CAD build for the part. Positions are in the model's coordinates, mm. Give positions to 0.01 mm unless a question says otherwise; leave off trailing zeros. Write each loop counter-clockwise with the first axis right and the second up, starting at its lowest first coordinate (ties: lowest second). Pieces come first, ordered by that corner, then holes. Notation, with made-up numbers: (44, -35) - (85, -35) arc R21 cw to (85, -14) - close; hole circle Ø10 at (87.25, 88). An arc over 180 degrees is marked (long way). Answer as a JSON object with one key per item and string values.
Autodesk Inventor part; units mm, degrees
ref_plane "XZ Plane" through (0, 0, 0) normal (0, 1, 0) x (-1, 0, 0)
ref_plane "XY Plane" through (0, 0, 0) normal (0, 0, 1) x (1, 0, 0)
sketch "Sketch1" plane through (0, 0, 0) normal (0, 1, 0) x (-1, 0, 0)
  line L0 (0, 0) -> (0, -399.562) construction
  line L1 (5, 0) -> (5, -399.562)
  line L2 (-5, -399.562) -> (-5, 0)
  arc A0 (5, 0) -> (-5, 0) centre (0, 0) ccw
  arc A1 (-5, -399.562) -> (5, -399.562) centre (0, -399.562) ccw
  circle A2 centre (0, -399.562) radius 1.65
  line L3 (0, -10) -> (0, -379.562) construction
  line L4 (-1.65, -10) -> (-1.65, -379.562)
  line L5 (1.65, -379.562) -> (1.65, -10)
  arc A3 (1.65, -10) -> (-1.65, -10) centre (0, -10) ccw
  arc A4 (-1.65, -379.562) -> (1.65, -379.562) centre (0, -379.562) ccw
  point P0 (0, -199.781)
  point P1 (0, -194.781)
  dimension "d1" = 3.3
  dimension "d2" = 10
  dimension "d3" = 399.562
  dimension "d16" = 3.3
  dimension "d17" = 20
  dimension "d18" = 10
extrude "Extrusion1" add sketch "Sketch1" along normal blind 6
sketch "Sketch2" plane through (0, 6, 0) normal (0, 1, 0) x (1, 0, 0)
  line L0 (-5, 399.562) -> (-5, 0)
  arc A0 (-5, 0) -> (5, 0) centre (0, 0) ccw
  line L1 (5, 0) -> (5, 399.562)
  arc A1 (5, 399.562) -> (-5, 399.562) centre (0, 399.562) ccw
  arc A2 (-1.65, 10) -> (1.65, 10) centre (0, 10) ccw
  line L2 (-1.65, 10) -> (-1.65, 379.562)
  arc A3 (1.65, 379.562) -> (-1.65, 379.562) centre (0, 379.562) ccw
  line L3 (1.65, 379.562) -> (1.65, 10)
  circle A4 centre (0, 399.562) radius 1.65
  line L4 (-5, 399.562) -> (-5, 0)
  line L5 (5, 0) -> (5, 399.562)
  circle A5 centre (0, 384.562) radius 5
  point P0 (-5, 384.562)
  point P1 (5, 384.562)
  dimension "d20" = 15
  dimension "d21" = 10
extrude "Extrusion2" add sketch "Sketch2" along normal blind 4 contours A1 L1 A5 L0 | A5 A3 | A3 A5
sketch "Sketch3" plane through (0, 0, 0) normal (0, -1, 0) x (1, 0, 0)
  line L0 (-5, -399.562) -> (-5, 0)
  arc A0 (-5, -399.562) -> (5, -399.562) centre (0, -399.562) ccw
  line L1 (5, 0) -> (5, -399.562)
  arc A1 (5, 0) -> (-5, 0) centre (0, 0) ccw
  arc A2 (1.65, -10) -> (-1.65, -10) centre (0, -10) ccw
  line L2 (1.65, -379.562) -> (1.65, -10)
  arc A3 (-1.65, -379.562) -> (1.65, -379.562) centre (0, -379.562) ccw
  line L3 (-1.65, -10) -> (-1.65, -379.562)
  circle A4 centre (0, -399.562) radius 1.65
  circle A5 centre (0, -384.562) radius 5
  point P0 (5, -384.562)
  point P1 (-5, -384.562)
  dimension "d24" = 10
  dimension "d25" = 15
extrude "Extrusion3" add sketch "Sketch3" along normal blind 4 contours L0 A5 L1 A0 | A5 A3 | A5 A3
extrude "Extrusion4" cut sketch "Sketch2" against normal blind 6 contours A1 L1 A5 L0
sketch "Sketch4" plane through (0, 0, 0) normal (0, 1, 0) x (1, 0, 0)
  line L0 (-5, 384.562) -> (-5, 399.562)
  arc A0 (5, 384.562) -> (-5, 384.562) centre (0, 384.562) ccw
  line L1 (5, 399.562) -> (5, 384.562)
  arc A1 (5, 399.562) -> (-5, 399.562) centre (0, 399.562) ccw
  circle A2 centre (0, 399.562) radius 1.65
  point P0 (0, 0)
extrude "Extrusion5" cut sketch "Sketch4" against normal blind 0.2
sketch "Sketch5" plane through (0, 6, 0) normal (0, -1, 0) x (1, 0, 0)
  line L0 (-5, -399.562) -> (-5, -384.562)
  arc A0 (-5, -399.562) -> (5, -399.562) centre (0, -399.562) ccw
  line L1 (5, -384.562) -> (5, -399.562)
  arc A1 (-5, -384.562) -> (5, -384.562) centre (0, -384.562) ccw
  circle A2 centre (0, -399.562) radius 1.65
  point P0 (0, 0)
extrude "Extrusion6" cut sketch "Sketch5" against normal blind 0.2
Item 1: Cut at B-B (x = 0). Give the cut face in (y, z), and give its area (3 significant figures).
Entries:
{"outline": "(-4, -404.56) - (-0.2, -404.56) - (-0.2, -401.21) - (-4, -401.21) - close; (-4, -397.91) - (-0.2, -397.91) - (-0.2, -389.56) - (6.2, -389.56) - (6.2, -397.91) - (10, -397.91) - (10, -379.56) - (6, -379.56) - (6, -381.21) - (0, -381.21) - (0, -379.56) - (-4, -379.56) - close; (0, -8.35) - (6, -8.35) - (6, 5) - (0, 5) - close; (6.2, -404.56) - (10, -404.56) - (10, -401.21) - (6.2, -401.21) - close", "area": "299 mm2"}
Item 2: Mould opens along Y. For faces 1 (the flat face through (0, -4, -392)), 2 (the flat face through (0, -0.2, -397)), 3 (the flat face through (2, 6, -187)), 4 (the flat face through (0, 6.2, -397)) say: +Y half, -Y half, draft (parallel to the pull), parting line (faces both ways), or undercut.
Entries:
{"face 1": "-Y half", "face 2": "undercut", "face 3": "+Y half", "face 4": "undercut"}
Item 3: Cut at C-C (y = 3.75). Give the cut face in (x, z).
Entries:
{"outline": "(-5, -384.56) arc R5 ccw to (5, -384.56) - (5, 0) arc R5 ccw to (-5, 0) - close; hole (-1.65, -379.56) arc R1.65 ccw to (1.65, -379.56) - (1.65, -10) arc R1.65 ccw to (-1.65, -10) - close"}
Item 4: Cut at A-A (z = -135.5). Give the cut face in (x, y), and give its area (3 significant figures).
Entries:
{"outline": "(-5, 0) - (-1.65, 0) - (-1.65, 6) - (-5, 6) - close; (1.65, 0) - (5, 0) - (5, 6) - (1.65, 6) - close", "area": "40.2 mm2"}
Item 5: Probe line 1 (Z direction, x = 0, y = 7.8); line 2 (X direction, y = 2, z = -243); line 3 (Z direction, x = -0.5, y = 5.25). List the from-to ranges inside material, lowest first. Write a range as from..to.
Entries:
{"line 1": "-404.56..-401.21, -397.91..-379.56", "line 2": "-5..-1.65, 1.65..5", "line 3": "-389.54..-381.13, -8.43..4.97"}
Item 6: Flat gauge pins, fed straight in: P1, Ø4, axis at x = -2.5, z = -169, coming from the +Y side; P2, Ø4, axis at x = -3, y = -0.5, coming from the +Z side. Where does each tip first touch, or does it go through?
Entries:
{"P1": "y = 6", "P2": "z = 4.89"}
